```python
from build123d import *

# Parameters (mm, degrees)
BASE_FLANGE1_DEPTH             = 104
EDGE_FLANGE1_STRIP_W           = 6
EDGE_FLANGE1_STRIP_H           = 1
EDGE_FLANGE1_STRIP_CUT_DEPTH   = 1202
EDGE_FLANGE1_RELIEF_W          = 6.5
EDGE_FLANGE1_RELIEF_H          = 0.5
EDGE_FLANGE1_RELIEF_CUT_DEPTH  = 1
EDGE_FLANGE1_DEPTH             = 1202
EDGE_FLANGE2_STRIP_W           = 6
EDGE_FLANGE2_STRIP_H           = 1
EDGE_FLANGE2_STRIP_CUT_DEPTH   = 1202
EDGE_FLANGE2_DEPTH             = 1202
EDGE_FLANGE3_STRIP_W           = 6
EDGE_FLANGE3_STRIP_H           = 1
EDGE_FLANGE3_STRIP_CUT_DEPTH   = 80
EDGE_FLANGE3_RELIEF_W          = 6.5
EDGE_FLANGE3_RELIEF_H          = 0.5
EDGE_FLANGE3_RELIEF_CUT_DEPTH  = 1
EDGE_FLANGE3_DEPTH             = 80
EDGE_FLANGE4_STRIP_W           = 6
EDGE_FLANGE4_STRIP_H           = 1
EDGE_FLANGE4_STRIP_CUT_DEPTH   = 80
EDGE_FLANGE4_DEPTH             = 80
EDGE_FLANGE5_STRIP_W           = 6
EDGE_FLANGE5_STRIP_H           = 1
EDGE_FLANGE5_STRIP_CUT_DEPTH   = 1158
EDGE_FLANGE5_RELIEF_W          = 6.5
EDGE_FLANGE5_RELIEF_H          = 0.5
EDGE_FLANGE5_RELIEF_CUT_DEPTH  = 1
EDGE_FLANGE5_DEPTH             = 1158
EDGE_FLANGE6_STRIP_W           = 6
EDGE_FLANGE6_STRIP_H           = 1
EDGE_FLANGE6_STRIP_CUT_DEPTH   = 80
EDGE_FLANGE6_RELIEF_W          = 6.5
EDGE_FLANGE6_RELIEF_H          = 0.5
EDGE_FLANGE6_RELIEF_CUT_DEPTH  = 1
EDGE_FLANGE6_DEPTH             = 80
SKETCH25_R                     = 3
CUT_EXTRUDE1_DEPTH             = 3
SKETCH26_R                     = 3
CUT_EXTRUDE2_DEPTH             = 3
CUT_EXTRUDE2_DIRECTION_2_REACH = 1234.559


# Sheet-metal steps are written as plain solids
with BuildPart() as part:
    # Sketch1 → Base-Flange1 (new body)
    with BuildSketch(Plane.XY):
        with BuildLine():
            Line((-621, -100), (-621, -15))
            ThreePointArc((-621, -15), (-616.606601718, -4.393398282), (-606, 0))
            Line((-606, 0), (606, 0))
            ThreePointArc((606, 0), (616.606601718, -4.393398282), (621, -15))
            Line((621, -15), (621, -100))
            Line((621, -100), (622, -100))
            Line((622, -100), (622, -15))
            ThreePointArc((622, -15), (617.313708499, -3.686291501), (606, 1))
            Line((606, 1), (-606, 1))
            ThreePointArc((-606, 1), (-617.313708499, -3.686291501), (-622, -15))
            Line((-622, -15), (-622, -100))
            Line((-622, -100), (-621, -100))
        make_face()
    extrude(amount=BASE_FLANGE1_DEPTH)

    # Edge-Flange1 strip (across the edge) → Edge-Flange1 strip cut (cut)
    with BuildSketch(Plane(origin=(-601, 0, 0), x_dir=(0, 0, 1), z_dir=(1, 0, 0))):
        with Locations((-2, -0.5)):
            Rectangle(EDGE_FLANGE1_STRIP_W, EDGE_FLANGE1_STRIP_H)
    extrude(amount=EDGE_FLANGE1_STRIP_CUT_DEPTH, mode=Mode.SUBTRACT)

    # Edge-Flange1 relief (on the sheet) → Edge-Flange1 relief cut (cut)
    with BuildSketch(Plane(origin=(-601, 0, 1), x_dir=(0, 0, 1), z_dir=(0, -1, 0))):
        with Locations((-2.75, 0.25)):
            Rectangle(EDGE_FLANGE1_RELIEF_W, EDGE_FLANGE1_RELIEF_H)
        with Locations((-2.75, -1202.25)):
            Rectangle(EDGE_FLANGE1_RELIEF_W, EDGE_FLANGE1_RELIEF_H)
    extrude(amount=-EDGE_FLANGE1_RELIEF_CUT_DEPTH, mode=Mode.SUBTRACT)

    # Edge-Flange1 section (across the edge) → Edge-Flange1 (add)
    with BuildSketch(Plane(origin=(-601, 0, 0), x_dir=(0, 0, 1), z_dir=(1, 0, 0))):
        with BuildLine():
            Line((-1, 1), (-1, 19))
            Line((-1, 19), (0, 19))
            Line((0, 19), (0, 1))
            ThreePointArc((0, 1), (0.292893219, 0.292893219), (1, 0))
            Line((1, 0), (1, -1))
            ThreePointArc((1, -1), (-0.414213562, -0.414213562), (-1, 1))
        make_face()
    extrude(amount=EDGE_FLANGE1_DEPTH)

    # Edge-Flange2 strip (across the edge) → Edge-Flange2 strip cut (cut)
    with BuildSketch(Plane(origin=(-601, -19, 0), x_dir=(0, 1, 0), z_dir=(1, 0, 0))):
        with Locations((-1, -0.5)):
            Rectangle(EDGE_FLANGE2_STRIP_W, EDGE_FLANGE2_STRIP_H)
    extrude(amount=EDGE_FLANGE2_STRIP_CUT_DEPTH, mode=Mode.SUBTRACT)

    # Edge-Flange2 section (across the edge) → Edge-Flange2 (add)
    with BuildSketch(Plane(origin=(-601, -19, 0), x_dir=(0, 1, 0), z_dir=(1, 0, 0))):
        with BuildLine():
            Line((0, 1), (0, 18))
            Line((0, 18), (1, 18))
            Line((1, 18), (1, 1))
            ThreePointArc((1, 1), (1.292893219, 0.292893219), (2, 0))
            Line((2, 0), (2, -1))
            ThreePointArc((2, -1), (0.585786438, -0.414213562), (0, 1))
        make_face()
    extrude(amount=EDGE_FLANGE2_DEPTH)

    # Edge-Flange3 strip (across the edge) → Edge-Flange3 strip cut (cut)
    with BuildSketch(Plane(origin=(-621, -100, 0), x_dir=(0, 0, 1), z_dir=(0, 1, 0))):
        with Locations((-2, -0.5)):
            Rectangle(EDGE_FLANGE3_STRIP_W, EDGE_FLANGE3_STRIP_H)
    edge_flange3_strip_cut = extrude(amount=EDGE_FLANGE3_STRIP_CUT_DEPTH, mode=Mode.SUBTRACT)

    # Edge-Flange3 relief (on the sheet) → Edge-Flange3 relief cut (cut)
    with BuildSketch(Plane(origin=(-621, -100, 1), x_dir=(0, 0, 1), z_dir=(1, 0, 0))):
        with Locations((-2.75, -80.25)):
            Rectangle(EDGE_FLANGE3_RELIEF_W, EDGE_FLANGE3_RELIEF_H)
    edge_flange3_relief_cut = extrude(amount=-EDGE_FLANGE3_RELIEF_CUT_DEPTH, mode=Mode.SUBTRACT)

    # Edge-Flange3 section (across the edge) → Edge-Flange3 (add)
    with BuildSketch(Plane(origin=(-621, -100, 0), x_dir=(0, 0, 1), z_dir=(0, 1, 0))):
        with BuildLine():
            Line((-1, 1), (-1, 19))
            Line((-1, 19), (0, 19))
            Line((0, 19), (0, 1))
            ThreePointArc((0, 1), (0.292893219, 0.292893219), (1, 0))
            Line((1, 0), (1, -1))
            ThreePointArc((1, -1), (-0.414213562, -0.414213562), (-1, 1))
        make_face()
    edge_flange3 = extrude(amount=EDGE_FLANGE3_DEPTH)

    # Edge-Flange4 strip (across the edge) → Edge-Flange4 strip cut (cut)
    with BuildSketch(Plane(origin=(-602, -100, 0), x_dir=(-1, 0, 0), z_dir=(0, 1, 0))):
        with Locations((-1, -0.5)):
            Rectangle(EDGE_FLANGE4_STRIP_W, EDGE_FLANGE4_STRIP_H)
    edge_flange4_strip_cut = extrude(amount=EDGE_FLANGE4_STRIP_CUT_DEPTH, mode=Mode.SUBTRACT)

    # Edge-Flange4 section (across the edge) → Edge-Flange4 (add)
    with BuildSketch(Plane(origin=(-602, -100, 0), x_dir=(-1, 0, 0), z_dir=(0, 1, 0))):
        with BuildLine():
            Line((0, 1), (0, 18))
            Line((0, 18), (1, 18))
            Line((1, 18), (1, 1))
            ThreePointArc((1, 1), (1.292893219, 0.292893219), (2, 0))
            Line((2, 0), (2, -1))
            ThreePointArc((2, -1), (0.585786438, -0.414213562), (0, 1))
        make_face()
    edge_flange4 = extrude(amount=EDGE_FLANGE4_DEPTH)

    # Mirror1: Edge-Flange3 strip cut, Edge-Flange3 relief cut, Edge-Flange3, Edge-Flange4 strip cut, Edge-Flange4 across plane
    add(edge_flange3_strip_cut.mirror(Plane(origin=(0, 0, 0), x_dir=(0, 0, 1), z_dir=(1, 0, 0))), mode=Mode.SUBTRACT)
    add(edge_flange3_relief_cut.mirror(Plane(origin=(0, 0, 0), x_dir=(0, 0, 1), z_dir=(1, 0, 0))), mode=Mode.SUBTRACT)
    add(edge_flange3.mirror(Plane(origin=(0, 0, 0), x_dir=(0, 0, 1), z_dir=(1, 0, 0))))
    add(edge_flange4_strip_cut.mirror(Plane(origin=(0, 0, 0), x_dir=(0, 0, 1), z_dir=(1, 0, 0))), mode=Mode.SUBTRACT)
    add(edge_flange4.mirror(Plane(origin=(0, 0, 0), x_dir=(0, 0, 1), z_dir=(1, 0, 0))))

    # Edge-Flange5 strip (across the edge) → Edge-Flange5 strip cut (cut)
    with BuildSketch(Plane(origin=(579, 0, 104), x_dir=(0, 0, -1), z_dir=(-1, 0, 0))):
        with Locations((-2, -0.5)):
            Rectangle(EDGE_FLANGE5_STRIP_W, EDGE_FLANGE5_STRIP_H)
    extrude(amount=EDGE_FLANGE5_STRIP_CUT_DEPTH, mode=Mode.SUBTRACT)

    # Edge-Flange5 relief (on the sheet) → Edge-Flange5 relief cut (cut)
    with BuildSketch(Plane(origin=(579, 0, 103), x_dir=(0, 0, -1), z_dir=(0, -1, 0))):
        with Locations((-2.75, 0.25)):
            Rectangle(EDGE_FLANGE5_RELIEF_W, EDGE_FLANGE5_RELIEF_H)
        with Locations((-2.75, -1158.25)):
            Rectangle(EDGE_FLANGE5_RELIEF_W, EDGE_FLANGE5_RELIEF_H)
    extrude(amount=-EDGE_FLANGE5_RELIEF_CUT_DEPTH, mode=Mode.SUBTRACT)

    # Edge-Flange5 section (across the edge) → Edge-Flange5 (add)
    with BuildSketch(Plane(origin=(579, 0, 104), x_dir=(0, 0, -1), z_dir=(-1, 0, 0))):
        with BuildLine():
            Line((-1, 1), (-1, 55))
            Line((-1, 55), (0, 55))
            Line((0, 55), (0, 1))
            ThreePointArc((0, 1), (0.292893219, 0.292893219), (1, 0))
            Line((1, 0), (1, -1))
            ThreePointArc((1, -1), (-0.414213562, -0.414213562), (-1, 1))
        make_face()
    extrude(amount=EDGE_FLANGE5_DEPTH)

    # Edge-Flange6 strip (across the edge) → Edge-Flange6 strip cut (cut)
    with BuildSketch(Plane(origin=(621, -100, 104), x_dir=(0, 0, -1), z_dir=(0, 1, 0))):
        with Locations((-2, -0.5)):
            Rectangle(EDGE_FLANGE6_STRIP_W, EDGE_FLANGE6_STRIP_H)
    edge_flange6_strip_cut = extrude(amount=EDGE_FLANGE6_STRIP_CUT_DEPTH, mode=Mode.SUBTRACT)

    # Edge-Flange6 relief (on the sheet) → Edge-Flange6 relief cut (cut)
    with BuildSketch(Plane(origin=(621, -100, 103), x_dir=(0, 0, -1), z_dir=(-1, 0, 0))):
        with Locations((-2.75, -80.25)):
            Rectangle(EDGE_FLANGE6_RELIEF_W, EDGE_FLANGE6_RELIEF_H)
    edge_flange6_relief_cut = extrude(amount=-EDGE_FLANGE6_RELIEF_CUT_DEPTH, mode=Mode.SUBTRACT)

    # Edge-Flange6 section (across the edge) → Edge-Flange6 (add)
    with BuildSketch(Plane(origin=(621, -100, 104), x_dir=(0, 0, -1), z_dir=(0, 1, 0))):
        with BuildLine():
            Line((-1, 1), (-1, 41))
            Line((-1, 41), (0, 41))
            Line((0, 41), (0, 1))
            ThreePointArc((0, 1), (0.292893219, 0.292893219), (1, 0))
            Line((1, 0), (1, -1))
            ThreePointArc((1, -1), (-0.414213562, -0.414213562), (-1, 1))
        make_face()
    edge_flange6 = extrude(amount=EDGE_FLANGE6_DEPTH)

    # Mirror2: Edge-Flange6 strip cut, Edge-Flange6 relief cut, Edge-Flange6 across plane
    add(edge_flange6_strip_cut.mirror(Plane(origin=(0, 0, 0), x_dir=(0, 0, 1), z_dir=(1, 0, 0))), mode=Mode.SUBTRACT)
    add(edge_flange6_relief_cut.mirror(Plane(origin=(0, 0, 0), x_dir=(0, 0, 1), z_dir=(1, 0, 0))), mode=Mode.SUBTRACT)
    add(edge_flange6.mirror(Plane(origin=(0, 0, 0), x_dir=(0, 0, 1), z_dir=(1, 0, 0))))

    # Sketch25 → Cut-Extrude1 (cut)
    with BuildSketch(Plane.XZ.offset(19)):
        with Locations(Location((-540, 12, 0), (0, 0, 270))):
            Circle(SKETCH25_R)
        with Locations(Location((-360, 12, 0), (0, 0, 270))):
            Circle(SKETCH25_R)
        with Locations(Location((-180, 12, 0), (0, 0, 270))):
            Circle(SKETCH25_R)
        with Locations(Location((0, 12, 0), (0, 0, 270))):
            Circle(SKETCH25_R)
        with Locations(Location((180, 12, 0), (0, 0, 270))):
            Circle(SKETCH25_R)
        with Locations(Location((360, 12, 0), (0, 0, 270))):
            Circle(SKETCH25_R)
        with Locations(Location((540, 12, 0), (0, 0, 270))):
            Circle(SKETCH25_R)
    extrude(amount=-CUT_EXTRUDE1_DEPTH, mode=Mode.SUBTRACT)

    # Sketch26 → Cut-Extrude2 (cut)
    with BuildSketch(Plane(origin=(-602, 0, 0), x_dir=(0, 0, -1), z_dir=(1, 0, 0))):
        with Locations((-12, -68)):
            Circle(SKETCH26_R)
    extrude(amount=-CUT_EXTRUDE2_DEPTH, mode=Mode.SUBTRACT)

    # Cut-Extrude2 direction 2: up to this face of the body (flat: up to its plane)
    cut_extrude2_direction_2_end = Plane(part.part.faces().sort_by_distance((603, -60, 9.5))[0])
    # Sketch26 → Cut-Extrude2 direction 2 (cut, up to the picked face)
    with BuildSketch(Plane(origin=(-602, 0, 0), x_dir=(0, 0, -1), z_dir=(1, 0, 0)), mode=Mode.PRIVATE) as cut_extrude2_direction_2_sk1:
        with Locations((-12, -68)):
            Circle(SKETCH26_R)
    cut_extrude2_direction_2_tool1 = split(extrude(cut_extrude2_direction_2_sk1.sketch, amount=CUT_EXTRUDE2_DIRECTION_2_REACH, mode=Mode.PRIVATE), bisect_by=cut_extrude2_direction_2_end, keep=Keep.BOTH, mode=Mode.PRIVATE)
    add(cut_extrude2_direction_2_tool1.solids().sort_by(Axis((-602, -68, 12), (1, 0, 0)))[0], mode=Mode.SUBTRACT)


solid = part.part
```
For this review, take the finished solid that the model builds, in its own axes (mm). A direction names the side the tool comes from. Coordinates: 2 decimals unless noted, no trailing zeros. Write each loop counter-clockwise with the first axis right and the second up, starting at its lowest first coordinate (ties: lowest second). Pieces come first, ordered by that corner, then holes. Notation, with made-up numbers: (67.5, 80) - (89.5, 80) arc R21 cw to (89.5, 102) - close; hole circle Ø6 at (35.25, 81). An arc over 180 degrees is marked (long way). Answer in a Markdown table with one row per item. Add a question column.
Q1. We need section C-C, the plane z = 50. State the section outline as (x, y) points.
Q2. We need section B-B, the plane y = -39. Count the separate pieces of the cut face and the enclosed holes in it, and give its area (3 significant figures).
Q3. Tool access review of faces 4 (the flat face through (617, -4, 0)), 5 (the flat face through (-8, 0, 51)), 6 (the flat face through (-617.1, -4.6, 0)), 7 (the flat face through (8, -28, 104)), 8 (the flat face through (-609, 0, 104)): name each direction out of +Z, -Z, +X, -X, +Y, -Y from which nothing blocks a thin tool from reaching the whole face with its end or side.
Q4. We need section A-A, the plane x = 509. State the section outline as (y, z) points, and give its area (3 significant figures).
Q5. For probe 1 along X at (y, z) = (-71, 10); probe 2 along Z at (x, y) = (-360, -18.8); probe 3 along Z at (x, y) = (289, -2.5), list the stretches that pass through material, from the lowest coordinate up.
Q6. For P1, Ø5.5, axis at x = 540, z = 12, coming from the -Y side; P2, Ø16.5, axis at x = 598, y = -6.5, coming from the +Z side; P3, Ø13.5, axis at x = -177, z = 11.5, coming from the -Y side, all flat-tipped, find the tip position at first contact; note any pin that passes through.
Q7. Draft analysis for pull direction Y (two halves, no side actions). For faces 1 (the flat face through (600, -61, 104)), 2 (the flat face through (-607.6, -20, -0.6)), 3 (the flat face through (8, 1, 51)), state which applies: +Y half, -Y half, draft (parallel to the pull), parting line (faces both ways), or undercut.
Answer list:
| question | item | result |
|---|---|---|
| 1 | outline | (-622, -100) - (-621, -100) - (-621, -15) arc R15 cw to (-606, 0) - (606, 0) arc R15 cw to (621, -15) - (621, -100) - (622, -100) - (622, -15) arc R16 ccw to (606, 1) - (-606, 1) arc R16 ccw to (-622, -15) - close |
| 2 | separate pieces | 3 |
| 2 | enclosed holes | 0 |
| 2 | area | 1,520 mm2 |
| 3 | face 4 | -Z, +X, +Y |
| 3 | face 5 | none |
| 3 | face 6 | -Z, -X, +Y |
| 3 | face 7 | -Y |
| 3 | face 8 | +Z, -X, +Y |
| 4 | outline | (-55, 104) - (-1, 104) arc R1 cw to (0, 103) - (0, 1) arc R1 cw to (-1, 0) - (-17, 0) arc R1 cw to (-18, 1) - (-18, 18) - (-19, 18) - (-19, 1) arc R2 ccw to (-17, -1) - (-1, -1) arc R2 ccw to (1, 1) - (1, 103) arc R2 ccw to (-1, 105) - (-55, 105) - close |
| 4 | area | 196 mm2 |
| 5 | probe 1 | x = -622 to -621, -603 to -602, 602 to 603, 621 to 622 |
| 5 | probe 2 | z = 0.13 to 9, 15 to 18, 104 to 105 |
| 5 | probe 3 | z = -1 to 0, 104 to 105 |
| 6 | P1 | stops at y = 0 |
| 6 | P2 | stops at z = 104 |
| 6 | P3 | stops at y = -19 |
| 7 | face 1 | draft |
| 7 | face 2 | undercut |
| 7 | face 3 | +Y half |
